```python
from build123d import *

# Parameters (mm, degrees)
F1_DEPTH = 25


with BuildPart() as f1:
    # F0 (on Front) → F1 (new body)
    with BuildSketch(Plane.XZ):
        with BuildLine():
            ThreePointArc((210.7900996534, -39.1419847991), (237.6177301096, -26.3390851309), (251.3977370138, 0))
            Line((251.3977370138, 0), (220.75, 0))
            ThreePointArc((220.75, 0), (216.6313755102, -12.4080557961), (205.9104965167, -19.8904130406))
            ThreePointArc((205.9104965167, -19.8904130406), (203.7307412614, -21.3576975777), (202, -23.3347639831))
            Line((202, -23.3347639831), (202, -34.6340773268))
            ThreePointArc((202, -34.6340773268), (205.8105086824, -38.0278448107), (210.7900996534, -39.1419847991))
        make_face()
        with BuildLine():
            ThreePointArc((202, -23.3347639831), (200.2850186662, -28.984420655), (202, -34.6340773268))
            Line((202, -34.6340773268), (202, -23.3347639831))
        make_face()
        with BuildLine():
            Line((25.3114801989, 24.2953589364), (21.0646269025, 0))
            Line((21.0646269025, 0), (154, 0))
            Line((154, 0), (160.5472754862, 0))
            ThreePointArc((160.5472754862, 0), (166.8205732831, 6.8086025808), (174.7224661833, 11.6326489056))
            Line((174.7224661833, 11.6326489056), (190.8394987814, 18.6184778493))
            ThreePointArc((190.8394987814, 18.6184778493), (191.7478739862, 19.038511398), (192.6754452712, 19.4142575966))
            ThreePointArc((192.6754452712, 19.4142575966), (211.8020758636, 17.0667368091), (220.75, 0))
            Line((220.75, 0), (251.3977370138, 0))
            ThreePointArc((251.3977370138, 0), (242.2377138986, 36.1766919921), (209.6012580564, 54.2742282063))
            Line((209.6012580564, 54.2742282063), (119.6315883608, 63.1246931609))
            Line((119.6315883608, 63.1246931609), (25.3114801989, 24.2953589364))
        make_face()
        with BuildLine():
            ThreePointArc((20.4400724491, -3.5729453221), (-1.7931810673, -20.6723729083), (-20.75, 0))
            Line((-20.75, 0), (-49.3885839036, 0))
            Line((-49.3885839036, 0), (-42.5576653039, -18.7677946067))
            Line((-42.5576653039, -18.7677946067), (-75.8785055961, -44.3357746251))
            Line((-75.8785055961, -44.3357746251), (-99.7378202288, -106.6764599215))
            Line((-99.7378202288, -106.6764599215), (155.289266195, -87.449753308))
            Line((155.289266195, -87.449753308), (155.289266195, -36.919753308))
            Line((155.289266195, -36.919753308), (154.7796214415, -22.3254370622))
            ThreePointArc((154.7796214415, -22.3254370622), (154.6339324313, -20.1651687544), (154.6285738509, -18))
            ThreePointArc((154.6285738509, -18), (156.2841628525, -8.5713012671), (160.5472754862, 0))
            Line((160.5472754862, 0), (154, 0))
            Line((154, 0), (21.0646269025, 0))
            Line((21.0646269025, 0), (20.4400724491, -3.5729453221))
        make_face()
        Polygon((-49.3885839036, 0), (-20.75, 0), (-23.7132952534, 33.8706197351), (-96.3537068285, 19.7507540773), (-97.3887999889, 0), (-60.7786662376, 0), (-49.7400883137, 0.9657504298), align=None)
        Polygon((-97.5574338221, -3.2177252221), (-60.7786662376, 0), (-97.3887999889, 0), align=None)
    extrude(amount=F1_DEPTH)


solid = f1.part
```
Here's how the part is built. I have some questions about the finished solid (model axes, mm). A direction names the side the tool comes from. Give positions to 0.01 mm unless a question says otherwise; leave off trailing zeros. Loops run counter-clockwise (first coordinate to the right, second up) from the corner with the lowest first, then second, coordinate; pieces in that order, holes last. Notation, with made-up numbers: M 27.5,75 L 72.5,75 A13 cw 72.5,89 Z; hole C -22,43.5 d2. An arc over 180 degrees is marked long. Return JSON: item names as keys, results as strings.
Item 1: Imagine slicing it at B-B on y = -10.75. List the corners of the cut face in (x, z) for me.
A:
{"outline": "M -99.74,-106.68 L 155.29,-87.45 L 155.29,-36.92 L 154.78,-22.33 A33.39 cw 174.72,11.63 L 190.84,18.62 A20.75 cw long 205.91,-19.89 A10.16 ccw 210.79,-39.14 A47 ccw 209.6,54.27 L 119.63,63.12 L 25.31,24.3 L 20.44,-3.57 A20.75 cw -20.75,0 L -23.71,33.87 L -96.35,19.75 L -97.56,-3.22 L -49.74,0.97 L -42.56,-18.77 L -75.88,-44.34 Z"}
Item 2: Thinking about a two-plate mould opening in Z: for faces 1 (the flat face through (74, -25, -21)), 2 (the flat face through (-59.53, -12.32, 26.91)), 3 (the flat face through (-87.64, -12.32, -75.07)), which applies, released by +Z, released by -Z, zero draft, split by the parting line, or undercut?
A:
{"face 1": "zero draft", "face 2": "released by +Z", "face 3": "undercut"}
Item 3: I'm going to push flat-ended pins straight in: pin 1 Ø5 at (x, z) = (128, 24) entering from +Y; pin 2 Ø10 at (x, y) = (-40.5, -10.5) entering from -Z; pin 3 Ø3 at (y, z) = (-4, 0) entering from +X; pin 4 Ø12 at (x, y) = (164.5, -21) entering from -Z. Where does each tip first touch, or does it pass through?
A:
{"pin 1": "stops at y = 0", "pin 2": "stops at z = -102.59", "pin 3": "stops at x = 251.62", "pin 4": "stops at z = -3.37"}
Item 4: On a 3-axis mill with a long thin cutter (end or side, diameter ignored), from which of +Z, -Z, +X, -X, +Y, -Y can I reach the whole of each face in a straight line? I mean faces 4 (the flat face through (-73.983, -12.325, -1.155)), 5 (the flat face through (73.13, -12.32, 43.98)), 6 (the flat face through (-58.98, -12.32, -31.37)), 7 (the flat face through (182.668, -12.325, 15.077)), 8 (the flat face through (165.246, -12.325, 58.638)). Say none if no direction works.
A:
{"face 4": "+Y, -Y", "face 5": "+Z, +Y, -Y", "face 6": "-X, +Y, -Y", "face 7": "-Z, +Y, -Y", "face 8": "+Z, +X, +Y, -Y"}
Item 5: Imagine slicing it at A-A on z = 30.5. List the corners of the cut face in (x, y) for me.
A:
{"outline": "M -41.05,-25 L -23.42,-25 L -23.42,0 L -41.05,0 Z; M 40.38,-25 L 245.99,-25 L 245.99,0 L 40.38,0 Z"}
Item 6: Imagine slicing it at C-C on x = 224.5. List the corners of the cut face in (y, z) for me.
A:
{"outline": "M -25,-35.26 L 0,-35.26 L 0,50.26 L -25,50.26 Z"}
Item 7: Imagine slicing it at D-D on z = 49. List the corners of the cut face in (x, y) for me.
A:
{"outline": "M 85.32,-25 L 227.06,-25 L 227.06,0 L 85.32,0 Z"}
Item 8: Please list where these lines run through material, in increasing order: line 1 (X direction, y = -4.75, z = -13.5); line 2 (X direction, y = -8.5, z = 16.5); line 3 (X direction, y = -8, z = -71).
A:
{"line 1": "x = -44.47 to -15.76, 15.76 to 155.07, 215.76 to 247.05", "line 2": "x = -96.52 to -22.19, 23.95 to 185.95, 212.58 to 251.13", "line 3": "x = -86.08 to 155.29"}
